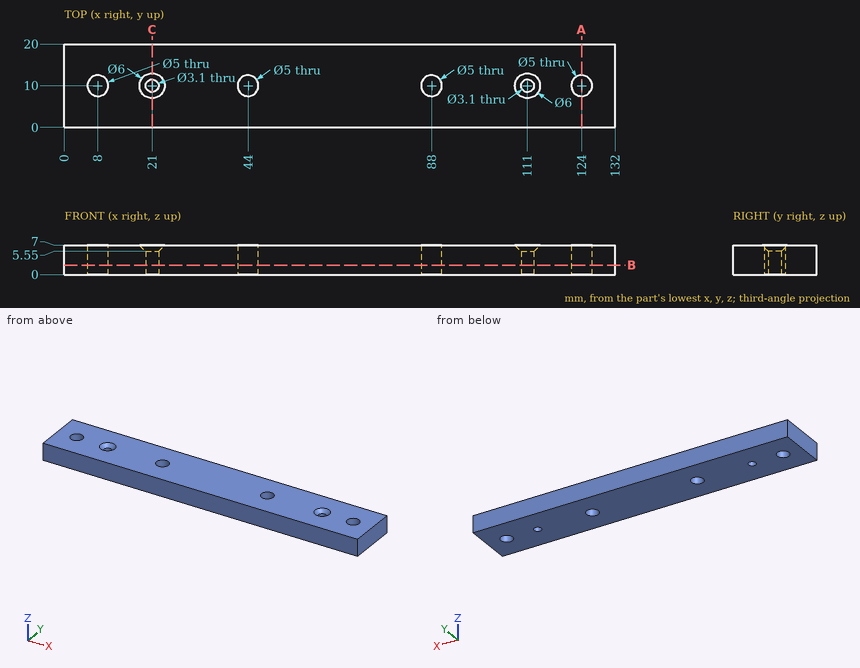
Could you check a few things on this drawing? It's one solid part, dimensions in mm from its lowest x, y, z. Coordinates: 2 decimals unless noted, no trailing zeros. Write each loop counter-clockwise with the first axis right and the second up, starting at its lowest first coordinate (ties: lowest second). Pieces come first, ordered by that corner, then holes. Notation, with made-up numbers: M -8.75,-38 L 19.25,-38 A14 cw 19.25,-26 Z; hole C 43,13.25 d4. An arc over 180 degrees is marked long. Answer as CSV lines item,"result". Start each with the question number.
Q1. I need wall thicknesses on probe 1 along Y at (x, z) = (124, 2); probe 2 along X at (y, z) = (7.75, 3). Which ranges of each line are inside material? Lowest first, please. Write a range as [from, to].
Q2. Will this pin go through, and if not, where does the flat tip stop? pin 1 Ø3 at (x, y) = (44, 10) entering from +Z.
Q3. Suppose I cut it at B-B, the plane z = 2.25. List the corners of the cut face in (x, y) for me.
Q4. Suppose I cut it at A-A, the plane x = 124. List the corners of the cut face in (y, z) for me.
Q5. Suppose I cut it at C-C, the plane x = 21. List the corners of the cut face in (y, z) for me.
Entries:
1,probe 1,"y = [0, 7.5], [12.5, 20]"
1,probe 2,"x = [0, 6.91], [9.09, 42.91], [45.09, 86.91], [89.09, 122.91], [125.09, 132]"
2,pin 1,"passes through"
3,outline,"M 0,0 L 132,0 L 132,20 L 0,20 Z; hole C 8,10 d5; hole C 21,10 d3.1; hole C 44,10 d5; hole C 88,10 d5; hole C 111,10 d3.1; hole C 124,10 d5"
4,outline,"M 0,0 L 7.5,0 L 7.5,7 L 0,7 Z; M 12.5,0 L 20,0 L 20,7 L 12.5,7 Z"
5,outline,"M 0,0 L 8.45,0 L 8.45,5.55 L 7,7 L 0,7 Z; M 11.55,0 L 20,0 L 20,7 L 13,7 L 11.55,5.55 Z"
